from build123d import *

# Parameters (mm, degrees)
F2_R     = 19.05
F3_DEPTH = 25.4
F4_SIZE  = 1.5875
F5_SIZE  = 1.5875


with BuildPart() as f1:
    # F0 (on Front) → F1 (revolve)
    with BuildSketch(Plane.XZ):
        Polygon((0, 107.95), (6.35, 107.95), (12.7, 107.95), (12.7, 120.65), (12.7, 133.35), (6.35, 133.35), (0, 133.35), (-12.741878, 133.35), (-12.741878, 107.95), (-6.35, 107.95), align=None)
        Polygon((-25.4, 19.05), (0, 19.05), (25.4, 19.05), (25.4, 38.1), (6.35, 38.1), (6.35, 107.95), (0, 107.95), (-6.35, 107.95), (-6.35, 38.1), (-25.4, 38.1), align=None)
    revolve(axis=Axis((38.116653, 0, 0), (1, 0, 0)))

    # F2 (on face) → F3 (cut)
    with BuildSketch(Plane.YZ.offset(6.35)):
        with Locations((-73.025, 0)):
            Circle(F2_R)
        with BuildLine():
            ThreePointArc((19.05, 73.025), (-13.470384, 86.495384), (0, 53.975))
            ThreePointArc((0, 53.975), (13.470384, 59.554616), (19.05, 73.025))
        make_face()
        with BuildLine():
            ThreePointArc((92.075, 0), (73.025, 19.05), (53.975, 0))
            ThreePointArc((53.975, 0), (73.025, -19.05), (92.075, 0))
        make_face()
        with BuildLine():
            ThreePointArc((19.05, -73.025), (13.470384, -59.554616), (0, -53.975))
            ThreePointArc((0, -53.975), (-13.470384, -86.495384), (19.05, -73.025))
        make_face()
    extrude(amount=-F3_DEPTH, mode=Mode.SUBTRACT)

    # F4
    f4_edges = [f1.edges().sort_by_distance(p)[0] for p in [
        (25.4, 0, -38.1),
        (25.4, 0, -19.05),
    ]]
    chamfer(f4_edges, length=F4_SIZE)

    # F5
    f5_edges = [f1.edges().sort_by_distance(p)[0] for p in [
        (-25.4, 0, -38.1),
        (-25.4, 0, -19.05),
    ]]
    chamfer(f5_edges, length=F5_SIZE)


solid = f1.part
Design review of the part built by this model. Coordinates are the model's own, in mm. A direction names the side the tool comes from. Coordinates: 2 decimals unless noted, no trailing zeros. Order: outer loops, then holes, each group sorted by start corner. A loop starts at its lowest first (then second) coordinate and runs counter-clockwise, first axis right, second up.
Item 1: For faces 5 (the cylindrical face through (0.33, 11.59, -15.12)), 6 (the cylindrical face through (-15.203, 23.183, -30.235)), 7 (the flat face through (6.35, -2, -46)), list the 3-axis set-ups (+Z, -Z, +X, -X, +Y, -Y) from which the entire face can be reached by the end or side of a thin tool; tool diameter is ignored.
Item 2: Take a section at D-D, the plane z = 0. Count the separate pieces of the cut face and the enclosed holes in it, then the cut area to 3 significant figures.
Item 3: The part is to be moulded in two halves that separate along Z. For faces 1 (the flat face through (12.7, 108, 11)), 2 (the cylindrical face through (14.959, 23.183, -30.235)), 3 (the cylindrical face through (-9.5, -72.96, -79.56)), 4 (the cylindrical face through (-0.199, -40.055, 127.192)), say which applies: pulls with the +Z half, pulls with the -Z half, needs draft (parallel to the pull), parting line crosses it, or undercut.
Item 4: Take a section at B-B, the plane y = 68. Write out the cut boundary in (x, z).
Item 5: For line 1 (Z direction, x = 10.5, y = 0); line 2 (X direction, y = -104, z = 38.5), list the stretches that pass through material, from the lowest coordinate up.
Item 6: For pin 1 Ø8 at (y, z) = (84.5, 27) entering from -X; pin 2 Ø23 at (y, z) = (73.025, 0) entering from +X; pin 3 Ø12 at (x, z) = (-0.5, 92.5) entering from -Y; pin 4 Ø4 at (x, y) = (9.5, -65) entering from +Z, all flat-tipped, find the tip position at first contact; note any pin that passes through.
Item 7: Take a section at C-C, the plane x = 20.5. Write out the cut boundary in (y, z).
Item 8: Take a section at A-A, the plane z = -84.5. Write out the cut boundary in (x, y).
The answers:
1. face 5: +X, -X
1. face 6: -X
1. face 7: +X
2. separate pieces: 4
2. enclosed holes: 0
2. area: 4,020 mm2
3. face 1: needs draft
3. face 2: undercut
3. face 3: undercut
3. face 4: parting line crosses it
4. outline: (-12.74, -114.71) - (12.7, -114.71) - (12.7, -83.84) - (6.35, -83.84) - (6.35, -18.38) - (-6.35, -18.38) - (-6.35, -83.84) - (-12.74, -83.84) - close; (-12.74, 83.84) - (-6.35, 83.84) - (-6.35, 18.38) - (6.35, 18.38) - (6.35, 83.84) - (12.7, 83.84) - (12.7, 114.71) - (-12.74, 114.71) - close
5. line 1: z = -133.35 to -107.95, -38.1 to -19.05, 19.05 to 38.1, 107.95 to 133.35
5. line 2: x = -12.74 to 12.7
6. pin 1: stops at x = -6.35
6. pin 2: passes through
6. pin 3: stops at y = -101.49
6. pin 4: stops at z = 117.53
7. outline: circle Ø76.2 at (0, 0); hole circle Ø38.1 at (0, 0)
8. outline: (-12.74, -103.16) - (12.7, -103.16) - (12.7, -67.18) - (6.35, -67.18) - (6.35, -15.21) - (-6.35, -15.21) - (-6.35, -67.18) - (-12.74, -67.18) - close; (-12.74, 67.18) - (-6.35, 67.18) - (-6.35, 15.21) - (6.35, 15.21) - (6.35, 67.18) - (12.7, 67.18) - (12.7, 103.16) - (-12.74, 103.16) - close
